Autodesk Inventor part; units mm, degrees
ref_plane "Start Plane" through (0, 0, 65.3224) normal (0, 0, 1) x (1, 0, 0)
ref_plane "End Plane" through (0, 0, 322.0408) normal (0, 0, 1) x (1, 0, 0)
ref_plane "Work Plane4" through (-14, 524.0032, 180.4251) normal (0, 0.19996, -0.9798041) x (1, 0, 0)
ref_plane "Start Plane" through (0, 0, 65.3224) normal (0, 0, 1) x (1, 0, 0)
ref_plane "End Plane" through (0, 0, 322.0408) normal (0, 0, 1) x (1, 0, 0)
sketch "Sketch" plane through (0, 0, 0) normal (0, 0, 1) x (1, 0, 0)
  line L0 (-20, -34) -> (-20, 34)
  line L1 (-14, 40) -> (14, 40)
  line L2 (20, 34) -> (20, -34)
  line L3 (14, -40) -> (-14, -40)
  arc A0 (-20, -34) -> (-14, -40) centre (-14, -34) ccw
  arc A1 (20, 34) -> (14, 40) centre (14, 34) ccw
  arc A2 (-14, 40) -> (-20, 34) centre (-14, 34) ccw
  arc A3 (14, -40) -> (20, -34) centre (14, -34) ccw
  arc A4 (-14, 37) -> (-17, 34) centre (-14, 34) ccw
  line L4 (-14, 37) -> (14, 37)
  arc A5 (17, 34) -> (14, 37) centre (14, 34) ccw
  line L5 (17, 34) -> (17, -34)
  arc A6 (14, -37) -> (17, -34) centre (14, -34) ccw
  line L6 (14, -37) -> (-14, -37)
  arc A7 (-17, -34) -> (-14, -37) centre (-14, -34) ccw
  line L7 (-17, -34) -> (-17, 34)
  line L8 (0, 57.7397) -> (0, -57.7397) construction
  line L9 (-29.7397, 0) -> (29.7397, 0) construction
  dimension "d7" = 6
  dimension "d9" = 40
  dimension "d11" = 80
  dimension "d12" = 3
  dimension "d15" = 20
  dimension "d16" = 40
extrude "Body" add sketch "Sketch" along normal up to surface (256.7184 mm away) from surface at 65.3224
sketch "Sketch3" plane through (0, 0, 0) normal (0, 0, 1) x (1, 0, 0)
  line L0 (0, 0) -> (10, 0)
ref_plane "Work Plane3" through (0, 0, 0) normal (0, -1, 0) x (1, 0, 0)
ref_plane "Work Plane4" through (-14, 524.0032, 180.4251) normal (0, 0.19996, -0.9798041) x (1, 0, 0)
split "Split1" plane through (-14, 524.0032, 180.4251) removes the side toward (0, 0.19996, -0.9798041)
sketch "Sketch4" plane through (0, 0, 0) normal (0, -1, 0) x (1, 0, 0)
  line L0 (-2, 65.3224) -> (12, 65.3224)
  line L1 (-2, 322.0408) -> (12, 322.0408)
  dimension "d18" = 256.7184
equation "\"d7\" = G_IR"
equation "\"d9\" = G_W"
equation "\"d11\" = G_H"
equation "\"d12\" = G_T"
equation "\"d15\" = 0.5 * d9"
equation "\"d16\" = 0.5 * d11"
equation "\"d3\" = G_L"
equation "\"G_W\" = 40"
equation "\"G_H\" = 80"
equation "\"G_T\" = 3"
equation "\"G_IR\" = 6"
equation "\"G_L\" = d18"
equation "\"G_OFFSET_START\" = -65.32245"
equation "\"d13\" = -G_OFFSET_START"
equation "\"d14\" = G_OFFSET_END + B_L"
equation "\"B_L\" = 402.04082"
properties part number "ISO 10799-2 - 80x40x3 - 256,72" material "Steel, Mild"
Check sheet for the modelled part. Datum: model origin and axes. Units: mm. A direction names the side the tool comes from. Coordinates: 2 decimals unless noted, no trailing zeros. Write each loop counter-clockwise with the first axis right and the second up, starting at its lowest first coordinate (ties: lowest second). Pieces come first, ordered by that corner, then holes. Notation, with made-up numbers: (43, 32.25) -> (81, 32.25) arc R5 ccw to (81, 36.25) -> close; hole circle Ø7 at (77, 69.25). An arc over 180 degrees is marked (long way). Use a Markdown table: item, result.
1. Tool access check on faces 1 (the flat face through (0, 40, 200)), 2 (the flat face through (0, -37, 192)). Record the directions out of +Z, -Z, +X, -X, +Y, -Y that give a thin tool (end or side, any length) a straight path to the whole face; none if there is none.
Reported:
| item | result |
|---|---|
| face 1 | +Z, -Z, +X, -X, +Y |
| face 2 | +Z, -Z |
2. Scan lines: line 1 along Y through (x, z) = (-10.5, 200); line 2 along X through (y, z) = (11, 242); line 3 along Y through (x, z) = (-16, 227). Record each from-to range of solid material in increasing order.
Reported:
| item | result |
|---|---|
| line 1 | y = -40 to -37, 37 to 40 |
| line 2 | x = -20 to -17, 17 to 20 |
| line 3 | y = -39.66 to -36.24, 36.24 to 39.66 |
3. Sectioned sample at C-C (y = 15). Enter the section's corners in (x, z).
Reported:
| item | result |
|---|---|
| outline | (-20, 76.55) -> (-17, 76.55) -> (-17, 322.04) -> (-20, 322.04) -> close; (17, 76.55) -> (20, 76.55) -> (20, 322.04) -> (17, 322.04) -> close |
4. Sectioned sample at A-A (x = -3). Enter the section's corners in (y, z), plus the area to 3 significant figures.
Reported:
| item | result |
|---|---|
| outline | (-40, 65.32) -> (-37, 65.93) -> (-37, 322.04) -> (-40, 322.04) -> close; (37, 81.04) -> (40, 81.65) -> (40, 322.04) -> (37, 322.04) -> close |
| area | 1,490 mm2 |
5. Sectioned sample at B-B (z = 168). Enter the section's corners in (x, y), plus the area to 3 significant figures.
Reported:
| item | result |
|---|---|
| outline | (-20, -34) arc R6 ccw to (-14, -40) -> (14, -40) arc R6 ccw to (20, -34) -> (20, 34) arc R6 ccw to (14, 40) -> (-14, 40) arc R6 ccw to (-20, 34) -> close; hole (-17, -34) arc R3 ccw to (-14, -37) -> (14, -37) arc R3 ccw to (17, -34) -> (17, 34) arc R3 ccw to (14, 37) -> (-14, 37) arc R3 ccw to (-17, 34) -> close |
| area | 661 mm2 |
6. Release check for a two-part mould opening along X. For faces 3 (the flat face through (-18, 0, 322.041)), 4 (the cylindrical face through (18.289, -38.196, 191.885)), 5 (the flat face through (-17, 0, 193)) record: pulls with the +X half, pulls with the -X half, needs draft (parallel to the pull), parting line crosses it, or undercut.
Reported:
| item | result |
|---|---|
| face 3 | needs draft |
| face 4 | pulls with the +X half |
| face 5 | undercut |
